from build123d import *

# Parameters (mm, degrees)
SKETCH1_R           = 2.6
BOSS_EXTRUDE1_DEPTH = 0.79375
CIRPATTERN1_COUNT   = 20


with BuildPart() as part:
    # Sketch1 → Boss-Extrude1 (new body)
    with BuildSketch(Plane(origin=(0, 0, 0), x_dir=(1, 0, 0), z_dir=(0, 1, 0))):
        with BuildLine():
            Line((-15.643446504, 98.76883406), (-13.77106769, 86.947099487))
            Line((-13.77106769, 86.947099487), (-13.2, 87.037547723))
            Line((-13.2, 87.037547723), (-13.2, 90.037547723))
            Line((-13.2, 90.037547723), (13.2, 90.037547723))
            Line((13.2, 90.037547723), (13.2, 87.037547723))
            Line((13.2, 87.037547723), (13.77106769, 86.947099487))
            Line((13.77106769, 86.947099487), (15.643446504, 98.76883406))
            ThreePointArc((15.643446504, 98.76883406), (0, 100), (-15.643446504, 98.76883406))
        make_face()
        with Locations(Location((0, 96.4, 0), (0, 0, 270))):
            Circle(SKETCH1_R, mode=Mode.SUBTRACT)
    extrude(amount=BOSS_EXTRUDE1_DEPTH)


with BuildPart() as cirpattern1_1:
    # CirPattern1: pattern copy
    add(part.part.rotate(Axis((0, 0, 0), (0, 1, 0)), 1 * 360 / CIRPATTERN1_COUNT))


with BuildPart() as cirpattern1_2:
    # CirPattern1: pattern copy
    add(part.part.rotate(Axis((0, 0, 0), (0, 1, 0)), 2 * 360 / CIRPATTERN1_COUNT))


with BuildPart() as cirpattern1_3:
    # CirPattern1: pattern copy
    add(part.part.rotate(Axis((0, 0, 0), (0, 1, 0)), 3 * 360 / CIRPATTERN1_COUNT))


with BuildPart() as cirpattern1_4:
    # CirPattern1: pattern copy
    add(part.part.rotate(Axis((0, 0, 0), (0, 1, 0)), 4 * 360 / CIRPATTERN1_COUNT))


with BuildPart() as cirpattern1_5:
    # CirPattern1: pattern copy
    add(part.part.rotate(Axis((0, 0, 0), (0, 1, 0)), 5 * 360 / CIRPATTERN1_COUNT))


with BuildPart() as cirpattern1_6:
    # CirPattern1: pattern copy
    add(part.part.rotate(Axis((0, 0, 0), (0, 1, 0)), 6 * 360 / CIRPATTERN1_COUNT))


with BuildPart() as cirpattern1_7:
    # CirPattern1: pattern copy
    add(part.part.rotate(Axis((0, 0, 0), (0, 1, 0)), 7 * 360 / CIRPATTERN1_COUNT))


with BuildPart() as cirpattern1_8:
    # CirPattern1: pattern copy
    add(part.part.rotate(Axis((0, 0, 0), (0, 1, 0)), 8 * 360 / CIRPATTERN1_COUNT))


with BuildPart() as cirpattern1_9:
    # CirPattern1: pattern copy
    add(part.part.rotate(Axis((0, 0, 0), (0, 1, 0)), 9 * 360 / CIRPATTERN1_COUNT))


with BuildPart() as cirpattern1_10:
    # CirPattern1: pattern copy
    add(part.part.rotate(Axis((0, 0, 0), (0, 1, 0)), 10 * 360 / CIRPATTERN1_COUNT))


with BuildPart() as cirpattern1_11:
    # CirPattern1: pattern copy
    add(part.part.rotate(Axis((0, 0, 0), (0, 1, 0)), 11 * 360 / CIRPATTERN1_COUNT))


with BuildPart() as cirpattern1_12:
    # CirPattern1: pattern copy
    add(part.part.rotate(Axis((0, 0, 0), (0, 1, 0)), 12 * 360 / CIRPATTERN1_COUNT))


with BuildPart() as cirpattern1_13:
    # CirPattern1: pattern copy
    add(part.part.rotate(Axis((0, 0, 0), (0, 1, 0)), 13 * 360 / CIRPATTERN1_COUNT))


with BuildPart() as cirpattern1_14:
    # CirPattern1: pattern copy
    add(part.part.rotate(Axis((0, 0, 0), (0, 1, 0)), 14 * 360 / CIRPATTERN1_COUNT))


with BuildPart() as cirpattern1_15:
    # CirPattern1: pattern copy
    add(part.part.rotate(Axis((0, 0, 0), (0, 1, 0)), 15 * 360 / CIRPATTERN1_COUNT))


with BuildPart() as cirpattern1_16:
    # CirPattern1: pattern copy
    add(part.part.rotate(Axis((0, 0, 0), (0, 1, 0)), 16 * 360 / CIRPATTERN1_COUNT))


with BuildPart() as cirpattern1_17:
    # CirPattern1: pattern copy
    add(part.part.rotate(Axis((0, 0, 0), (0, 1, 0)), 17 * 360 / CIRPATTERN1_COUNT))


with BuildPart() as cirpattern1_18:
    # CirPattern1: pattern copy
    add(part.part.rotate(Axis((0, 0, 0), (0, 1, 0)), 18 * 360 / CIRPATTERN1_COUNT))


with BuildPart() as cirpattern1_19:
    # CirPattern1: pattern copy
    add(part.part.rotate(Axis((0, 0, 0), (0, 1, 0)), 19 * 360 / CIRPATTERN1_COUNT))

    # Combine1: union CirPattern1_18, CirPattern1_17, CirPattern1_16, CirPattern1_15, CirPattern1_14, CirPattern1_13, CirPattern1_12, CirPattern1_11, CirPattern1_10, CirPattern1_9, CirPattern1_8, CirPattern1_7, CirPattern1_6, CirPattern1_5, CirPattern1_4, CirPattern1_3, CirPattern1_2, CirPattern1_1, part
    add(cirpattern1_18.part)
    add(cirpattern1_17.part)
    add(cirpattern1_16.part)
    add(cirpattern1_15.part)
    add(cirpattern1_14.part)
    add(cirpattern1_13.part)
    add(cirpattern1_12.part)
    add(cirpattern1_11.part)
    add(cirpattern1_10.part)
    add(cirpattern1_9.part)
    add(cirpattern1_8.part)
    add(cirpattern1_7.part)
    add(cirpattern1_6.part)
    add(cirpattern1_5.part)
    add(cirpattern1_4.part)
    add(cirpattern1_3.part)
    add(cirpattern1_2.part)
    add(cirpattern1_1.part)
    add(part.part)


solid = cirpattern1_19.part
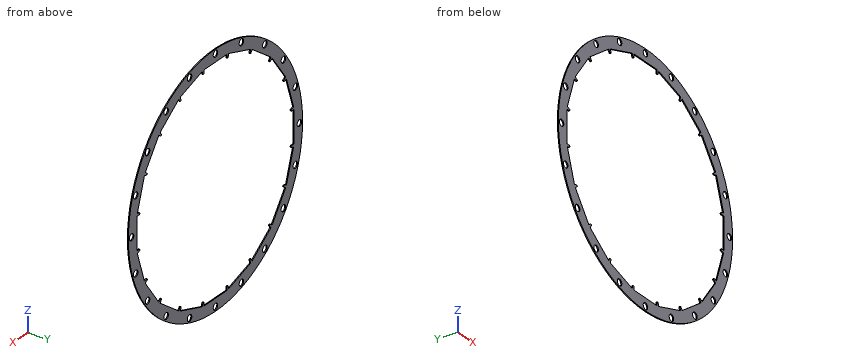
Verification items for the finished model (mm, model axes). Coordinates: 2 decimals unless noted, no trailing zeros. Write each loop counter-clockwise with the first axis right and the second up, starting at its lowest first coordinate (ties: lowest second). Pieces come first, ordered by that corner, then holes. Notation, with made-up numbers: (49.5, -22) - (57.5, -22) arc R16 cw to (57.5, -10) - close; hole circle Ø2 at (-28.5, 82.25). An arc over 180 degrees is marked (long way). Answer as a JSON object with one key per item and string values.
(1) Cross-section at B-B on z = 8.5. Record the cut outline in (x, y), plus the area to 3 significant figures.
Report:
{"outline": "(-99.64, 0) - (-90.04, 0) - (-90.04, 0.79) - (-99.64, 0.79) - close; (90.04, 0) - (99.64, 0) - (99.64, 0.79) - (90.04, 0.79) - close", "area": "15.2 mm^2"}
(2) Cross-section at C-C on y = 0.15. Give the number of separate pieces and of enclosed holes in the cut face, plus the area to 3 significant figures.
Report:
{"separate pieces": "1", "enclosed holes": "21", "area": "5,410 mm^2"}
(3) Cross-section at D-D on z = 48. Record the cut outline in (x, y).
Report:
{"outline": "(-87.73, 0) - (-76.42, 0) - (-76.42, 0.79) - (-87.73, 0.79) - close; (76.42, 0) - (87.73, 0) - (87.73, 0.79) - (76.42, 0.79) - close"}
(4) Thickness scan on line 1 along X through (y, z) = (0.4, 91.5); line 2 along Z through (x, y) = (-5, 0.65); line 3 along X through (y, z) = (0.45, -34.5). Record the ranges inside material, lowest first.
Report:
{"line 1": "-40.35 to -32.38, -27.2 to 27.2, 32.38 to 40.35", "line 2": "-99.87 to -90.04, 90.04 to 99.87", "line 3": "-93.86 to -83.46, 83.46 to 93.86"}
(5) Cross-section at A-A on x = 0. Record the cut outline in (y, z).
Report:
{"outline": "(0, -100) - (0.79, -100) - (0.79, -99) - (0, -99) - close; (0, -93.8) - (0.79, -93.8) - (0.79, -90.04) - (0, -90.04) - close; (0, 90.04) - (0.79, 90.04) - (0.79, 93.8) - (0, 93.8) - close; (0, 99) - (0.79, 99) - (0.79, 100) - (0, 100) - close"}
